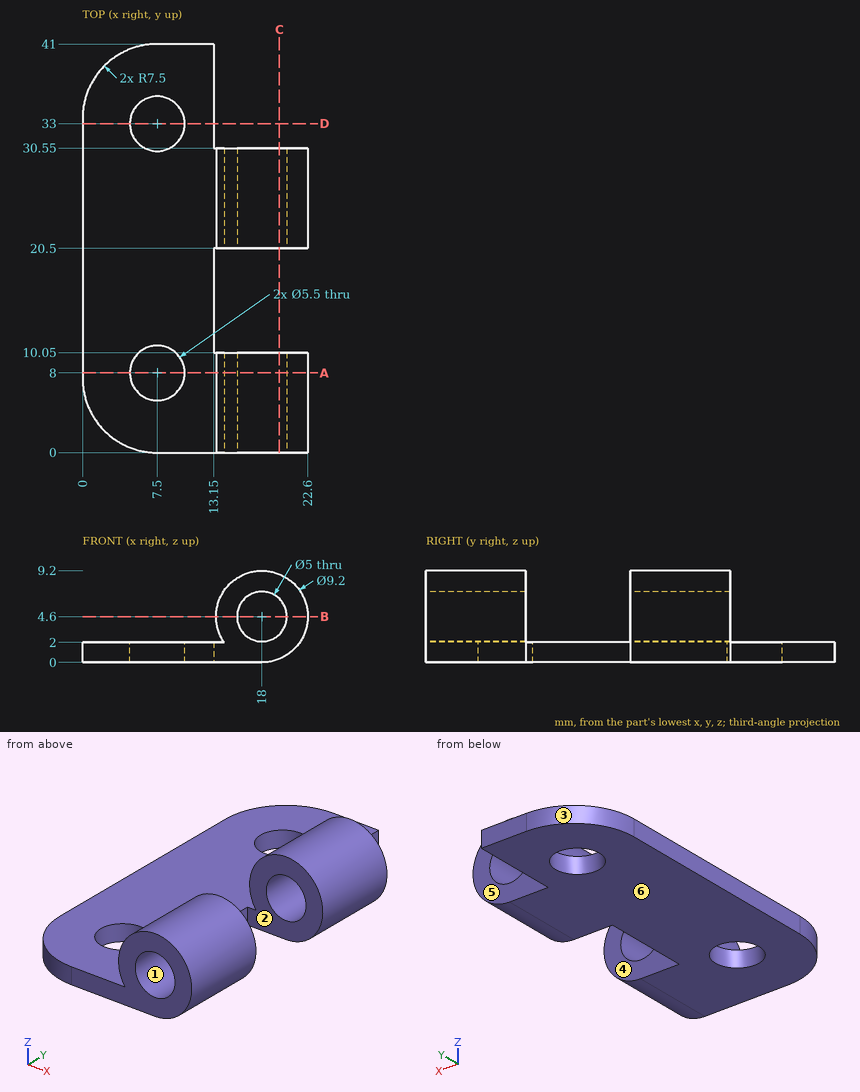
Geometry check sheet. Reference: drawing and pictorial views, mm from the part's lowest x, y, z. A direction names the side the tool comes from. Give positions to 0.01 mm unless a question says otherwise; leave off trailing zeros. Write each loop counter-clockwise with the first axis right and the second up, starting at its lowest first coordinate (ties: lowest second). Pieces come first, ordered by that corner, then holes. Notation, with made-up numbers: (-28, 19.25) - (21, 19.25) arc R8 ccw to (21, 33.25) - close; hole circle Ø11 at (-6.5, 84). An arc over 180 degrees is marked (long way). Use a Markdown table: item, result.
Q1. Set-up check for the marked faces 5 and 6: record each of +Z, -Z, +X, -X, +Y, -Y from which the full face is reachable in a straight line by a thin tool's end or side.
Computed:
| item | result |
|---|---|
| face 5 | +Z, -Z, +X, +Y |
| face 6 | -Z, +X, -X, +Y, -Y |
Q2. Section check D-D, the plane y = 33. Enter the section's corners in (x, z).
Computed:
| item | result |
|---|---|
| outline | (0, 0) - (4.75, 0) - (4.75, 2) - (0, 2) - close; (10.25, 0) - (13.15, 0) - (13.15, 2) - (10.25, 2) - close |
Q3. Go/stop test with flat-tipped pins: P1, Ø3, axis at x = 18, z = 4.6, coming from the +Y side; P2, Ø4.5, axis at x = 5, y = 15.5, coming from the +Z side; P3, Ø4.5, axis at x = 20, z = 6.5, coming from the +Y side; P4, Ø0.6, axis at y = 38, z = 1.5, coming from the +X side. Record where each tip stops, or that it passes through.
Computed:
| item | result |
|---|---|
| P1 | passes through |
| P2 | stops at z = 2 |
| P3 | stops at y = 30.55 |
| P4 | stops at x = 13.15 |
Q4. Section check A-A, the plane y = 8. Enter the section's corners in (x, z), then the cut area to 3 significant figures.
Computed:
| item | result |
|---|---|
| outline | (0, 0) - (4.75, 0) - (4.75, 2) - (0, 2) - close; (10.25, 0) - (18, 0) arc R4.6 ccw (long way) to (14.21, 2) - (10.25, 2) - close; hole circle Ø5 at (18, 4.6) |
| area | 66.5 mm² |
Q5. Draft check along Y on the marked faces 1, 2, 3 and 4. Enter one of: pulls with the +Y half, pulls with the -Y half, needs draft (parallel to the pull), parting line crosses it, or undercut.
Computed:
| item | result |
|---|---|
| face 1 | needs draft |
| face 2 | undercut |
| face 3 | pulls with the +Y half |
| face 4 | undercut |
Q6. Section check B-B, the plane z = 4.6. Enter the section's corners in (x, y), then the cut area to 3 significant figures.
Computed:
| item | result |
|---|---|
| outline | (13.4, 0) - (15.5, 0) - (15.5, 10.05) - (13.4, 10.05) - close; (13.4, 20.5) - (15.5, 20.5) - (15.5, 30.55) - (13.4, 30.55) - close; (20.5, 0) - (22.6, 0) - (22.6, 10.05) - (20.5, 10.05) - close; (20.5, 20.5) - (22.6, 20.5) - (22.6, 30.55) - (20.5, 30.55) - close |
| area | 84.4 mm² |
Q7. Thickness scan on L1, parallel to X at y = 9, z = 4.5; L2, parallel to Z at x = 18, y = 23.25; L3, parallel to Y at x = 21.5, z = 6. Record the ranges inside material, lowest first. Write a range as [from, to].
Computed:
| item | result |
|---|---|
| L1 | x = [13.4, 15.5], [20.5, 22.6] |
| L2 | z = [0, 2.1], [7.1, 9.2] |
| L3 | y = [0, 10.05], [20.5, 30.55] |
Q8. Section check C-C, the plane x = 19.75. Enter the section's corners in (y, z).
Computed:
| item | result |
|---|---|
| outline | (0, 0.35) - (10.05, 0.35) - (10.05, 2.81) - (0, 2.81) - close; (0, 6.39) - (10.05, 6.39) - (10.05, 8.85) - (0, 8.85) - close; (20.5, 0.35) - (30.55, 0.35) - (30.55, 2.81) - (20.5, 2.81) - close; (20.5, 6.39) - (30.55, 6.39) - (30.55, 8.85) - (20.5, 8.85) - close |
